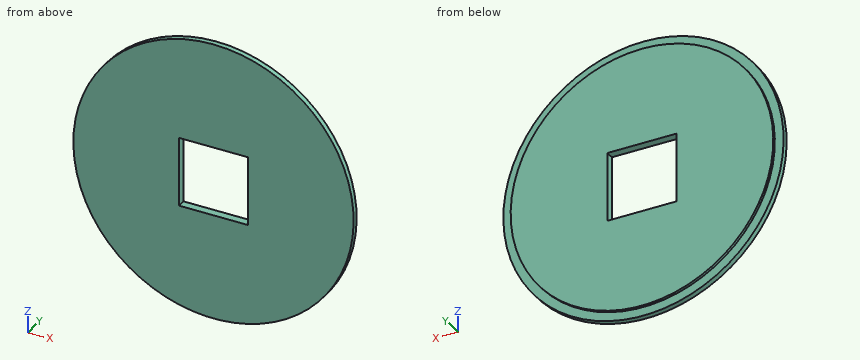
```python
from build123d import *

# Parameters (mm, degrees)
SKETCH2_W          = 50
SKETCH2_H          = 50
CUT_EXTRUDE1_DEPTH = 10


with BuildPart() as part:
    # Sketch1 → Revolve1 (revolve)
    with BuildSketch(Plane.XY, mode=Mode.PRIVATE) as revolve1_sk:
        Polygon((0, 0), (-101.15, 0), (-101.15, 4), (-94.8, 4), (-94.8, 6), (0, 6), align=None)
    revolve(revolve1_sk.sketch.rotate(Axis((0, 6, 0), (0, -1, 0)), 270), axis=Axis((0, 6, 0), (0, -1, 0)))

    # Sketch2 → Cut-Extrude1 (cut)
    with BuildSketch(Plane(origin=(0, 0, 0), x_dir=(1, 0, 0), z_dir=(0, 1, 0))):
        Rectangle(SKETCH2_W, SKETCH2_H)
    extrude(amount=CUT_EXTRUDE1_DEPTH, mode=Mode.SUBTRACT)


solid = part.part
```
Source: CAD feature listing. Evaluate the final solid. Frame: model axes, mm. Coordinates: 2 decimals unless noted, no trailing zeros. Loops run counter-clockwise (first coordinate to the right, second up) from the corner with the lowest first, then second, coordinate; pieces in that order, holes last. Notation, with made-up numbers: M -28.5,19 L 20.5,19 A20 ccw 20.5,38 Z; hole C 58.25,58.5 d10. An arc over 180 degrees is marked long. Put each result on its own line as item: value. Start each with the question number.
1) Cut plane D-D on x = -55. Return the cut outline in (y, z).
2) Contact query for flat-ended pins moving along their axis: pin 1 Ø3 at (y, z) = (4.5, 9.5) entering from +X; pin 2 Ø5 at (x, z) = (-23, -8) entering from -Y; pin 3 Ø2 at (x, y) = (30, 1.5) entering from +Z; pin 4 Ø2 at (x, y) = (52.5, 2) entering from +Z. Output: stop coordinate, or through.
3) Cut plane C-C on y = 1.7. Return the cut outline in (x, z), then the cut area to 3 significant figures.
4) Cut plane A-A on x = 0. Return the cut outline in (y, z), then the cut area to 3 significant figures.
5) Ray query, L1, parallel to Z at x = 10, y = 3.2; L2, parallel to Y at x = -82, z = -57.5; L3, parallel to Z at x = 3.5, y = 1.7. Return the intervals inside material, ascending. Write a range as from..to.
6) Cut plane B-B on z = 0. Return the cut outline in (x, y).
The answers:
1. outline: M 0,-84.89 L 4,-84.89 L 4,-77.21 L 6,-77.21 L 6,77.21 L 4,77.21 L 4,84.89 L 0,84.89 Z
2. pin 1: stops at x = 100.83
2. pin 2: stops at y = 0
2. pin 3: stops at z = 96.9
2. pin 4: stops at z = 87.06
3. outline: C 0,0 d202.3; hole M -25,-25 L 25,-25 L 25,25 L -25,25 Z
3. area: 29,600 mm²
4. outline: M 0,-101.15 L 4,-101.15 L 4,-94.8 L 6,-94.8 L 6,-25 L 0,-25 Z; M 0,25 L 6,25 L 6,94.8 L 4,94.8 L 4,101.15 L 0,101.15 Z
4. area: 888 mm²
5. L1: z = -100.65..-25, 25..100.65
5. L2: y = 0..4
5. L3: z = -101.09..-25, 25..101.09
6. outline: M -101.15,0 L -25,0 L -25,6 L -94.8,6 L -94.8,4 L -101.15,4 Z; M 25,0 L 101.15,0 L 101.15,4 L 94.8,4 L 94.8,6 L 25,6 Z
